Input: part model. Units: mm. Frame: model coordinates. A direction names the side the tool comes from. Round coordinates to 2 decimals unless told otherwise and drop trailing zeros. Loops run counter-clockwise (first coordinate to the right, second up) from the corner with the lowest first, then second, coordinate; pieces in that order, holes last. Notation, with made-up numbers: (11, 50) -> (59, 50) arc R28 ccw to (59, 85) -> close; hole circle Ø11 at (28, -6). An arc over 180 degrees is marked (long way). Answer as a JSON object with one key per item and string values. Group by question number.
Item 1: Section query A-A on y = -12.5. Return loops of the section in (x, z), and give its area (3 significant figures).
Item 2: Material intervals for line 1 (X direction, y = -4.75, z = -2.5); line 2 (X direction, y = -2, z = 18); line 3 (X direction, y = -20.75, z = 3.5), sorted ascending. Write a range as [from, to].
Item 3: Pin query (flat end, axial travel): pin 1 (2 mm diameter, centred on x = 3.5, y = -5, fed in from +Z); pin 2 (1.5 mm diameter, centred on x = 4.5, y = -26.5, fed in from -Z); pin 3 (5 mm diameter, centred on x = 68.5, y = -24.5, fed in from +Z); pin 4 (1 mm diameter, centred on x = -13, z = 8, fed in from +Y). Return the tip coordinate at first contact, or that it passes through.
Item 4: Draft query along X for faces 4 (the flat face through (1, -30, 7)), 5 (the flat face through (-59.634, -14.79, 9.77)). Return one class per face: released by +X, released by -X, zero draft, split by the parting line, or undercut.
Item 5: Section query D-D on x = -25. Return loops of the section in (y, z).
Item 6: Section query B-B on x = 75. Return loops of the section in (y, z).
Item 7: Set-up query: faces 1 (the flat face through (26, -15, 11.217)), 2 (the flat face through (-24.995, -14.79, 10.228)), 3 (the flat face through (1, 0, 7)). Return all of +Z, -Z, +X, -X, +Y, -Y with unobstructed straight access to the full face (end or side cutting, diameter ignored); none if empty.
Item 8: Section query C-C on z = 14.5. Return loops of the section in (x, y).
from build123d import *

# Parameters (mm, degrees)
F1_DEPTH = 30


with BuildPart() as f1:
    # F0 (on Front) → F1 (new body)
    with BuildSketch(Plane.XZ):
        with BuildLine():
            ThreePointArc((-14.7189177922, -12.0731056636), (-12.8233398948, -6.168347743), (-12.1823502003, 0))
            ThreePointArc((-12.1823502003, 0), (-12.7313900211, 5.7132254045), (-14.3584131685, 11.2173315922))
            ThreePointArc((-14.3584131685, 11.2173315922), (-72.178757015, 0.4643040074), (-14.7189177922, -12.0731056636))
        make_face()
        Polygon((-30.7383209178, 20.0591008551), (-19.0886446415, 0.1187303472), (-30.532673924, -19.9403705079), (-53.6263794829, -20.0591008551), (-65.2760557592, -0.1187303472), (-53.8320264766, 19.9403705079), align=None, mode=Mode.SUBTRACT)
        with BuildLine():
            ThreePointArc((-14.3584131685, 11.2173315922), (-12.7313900211, 5.7132254045), (-12.1823502003, 0))
            ThreePointArc((-12.1823502003, 0), (-12.8233398948, -6.168347743), (-14.7189177922, -12.0731056636))
            Line((-14.7189177922, -12.0731056636), (64.2681791355, -10.6453385498))
            ThreePointArc((64.2681791355, -10.6453385498), (61.2026273995, 0.3415440484), (64.6415868315, 11.2173315922))
            Line((64.6415868315, 11.2173315922), (-14.3584131685, 11.2173315922))
        make_face()
        with BuildLine():
            ThreePointArc((-5.1515232772, -4.3269232847), (-7.3021761652, 0.6730767153), (-5.1515232772, 5.6730767153))
            Line((-5.1515232772, 5.6730767153), (53.4061715007, 5.6730767153))
            ThreePointArc((53.4061715007, 5.6730767153), (55.808235454, 0.6730767153), (53.4061715007, -4.3269232847))
            Line((53.4061715007, -4.3269232847), (-5.1515232772, -4.3269232847))
        make_face(mode=Mode.SUBTRACT)
        with BuildLine():
            ThreePointArc((101.1997108784, 0), (87.0664612166, 19.1201788817), (64.6415868315, 11.2173315922))
            ThreePointArc((64.6415868315, 11.2173315922), (61.2026273995, 0.3415440484), (64.2681791355, -10.6453385498))
            ThreePointArc((64.2681791355, -10.6453385498), (86.7390865265, -19.2175783445), (101.1997108784, 0))
        make_face()
        Polygon((87.223782972, 17.5351066588), (99.7381289824, -0.3105870635), (86.6330112708, -17.7270600205), (66.0192570879, -10.6453385498), (66.1971306066, -0.0283681482), (66.3843740788, 11.147878975), align=None, mode=Mode.SUBTRACT)
    extrude(amount=F1_DEPTH)


solid = f1.part
Solved:
{
 "1": {"outline": "(-14.72, -12.07) -> (64.27, -10.65) arc R20 ccw (long way) to (64.64, 11.22) -> (-14.36, 11.22) arc R30 ccw (long way) to start; hole (-65.28, -0.12) -> (-53.63, -20.06) -> (-30.53, -19.94) -> (-19.09, 0.12) -> (-30.74, 20.06) -> (-53.83, 19.94) -> close; hole (-5.15, -4.33) -> (53.41, -4.33) arc R6.4 ccw to (53.41, 5.67) -> (-5.15, 5.67) arc R6.89 ccw to start; hole (66.02, -10.65) -> (86.63, -17.73) -> (99.74, -0.31) -> (87.22, 17.54) -> (66.38, 11.15) -> close", "area": "2,960 mm²"},
 "2": {"line 1": "[-72.08, -63.88], [-20.58, -6.53], [54.97, 66.16], [98.09, 101.04]", "line 2": "[-66.18, -54.94], [-29.54, -18.18], [72.48, 89.92]", "line 3": "[-71.98, -63.21], [-21.06, -6.7], [55.15, 66.26], [97.07, 100.89]"},
 "3": {"pin 1": "z = 11.22", "pin 2": "z = -11.74", "pin 3": "z = 17.2", "pin 4": "y = 0"},
 "4": {"face 4": "zero draft", "face 5": "undercut"},
 "5": {"outline": "(-30, -24.59) -> (0, -24.59) -> (0, -10.24) -> (-30, -10.24) -> close; (-30, 10.24) -> (0, 10.24) -> (0, 24.59) -> (-30, 24.59) -> close"},
 "6": {"outline": "(-30, -19.01) -> (0, -19.01) -> (0, -13.73) -> (-30, -13.73) -> close; (-30, 13.79) -> (0, 13.79) -> (0, 19.01) -> (-30, 19.01) -> close"},
 "7": {"face 1": "+Z, +Y, -Y", "face 2": "+Y, -Y", "face 3": "+Z, -Z, +X, -X, +Y"},
 "8": {"outline": "(-68.45, -30) -> (-56.94, -30) -> (-56.94, 0) -> (-68.45, 0) -> close; (-27.49, -30) -> (-15.92, -30) -> (-15.92, 0) -> (-27.49, 0) -> close; (67.42, -30) -> (77.32, -30) -> (77.32, 0) -> (67.42, 0) -> close; (89.35, -30) -> (94.97, -30) -> (94.97, 0) -> (89.35, 0) -> close"}
}
